Geometry: final body of the model. Coordinates: model frame, mm. Face numbers are marked on the shaded views. A direction names the side the tool comes from. Coordinates: 2 decimals unless noted, no trailing zeros. Write each loop counter-clockwise with the first axis right and the second up, starting at its lowest first coordinate (ties: lowest second). Pieces come first, ordered by that corner, then holes. Notation, with made-up numbers: (81.25, 69) - (117.25, 69) arc R15 ccw to (117.25, 83) - close; hole circle Ø2 at (33.25, -34.5). An arc over 180 degrees is marked (long way). Put each result on its own line as item: value.
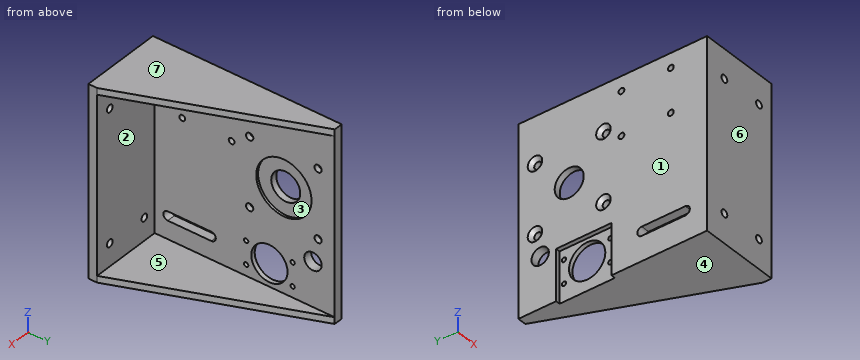
```python
from build123d import *

# Parameters (mm, degrees)
SKETCH1_W                  = 130
SKETCH1_H                  = 130
BOSS_EXTRUDE1_DEPTH        = 6
SKETCH2_W                  = 130
SKETCH2_H                  = 6
BOSS_EXTRUDE2_DEPTH        = 50
BOSS_EXTRUDE3_DEPTH        = 4.5
BOSS_EXTRUDE4_DEPTH        = 4.5
SKETCH5_R                  = 19.05
CUT_EXTRUDE1_DEPTH         = 1.6
SKETCH6_R                  = 10
CUT_EXTRUDE2_DEPTH         = 191.951721647
SKETCH7_R                  = 2.5
CUT_EXTRUDE3_DEPTH         = 193.187408537
SKETCH8_R                  = 12.5
SKETCH8_R_2                = 1.5
ENCODER_MOUNTING_DEPTH     = 193.187408537
SKETCH9_W                  = 35
SKETCH9_H                  = 38
SQR_SLOT_FRO_ENCODER_DEPTH = 3
SKETCH10_R                 = 6
CUT_EXTRUDE6_DEPTH         = 193.187408537
SKETCH12_R                 = 2
CUT_EXTRUDE8_DEPTH         = 193.187408537
CHAMFER1_SIZE              = 2.5
SKETCH14_R                 = 2.5
CUT_EXTRUDE10_DEPTH        = 193.187408537
CUT_EXTRUDE11_DEPTH        = 193.187408537


with BuildPart() as part:
    # Sketch1 → Boss-Extrude1 (new body)
    with BuildSketch(Plane(origin=(0, 0, 0), x_dir=(0, 0, -1), z_dir=(1, 0, 0))):
        with Locations((65, 65)):
            Rectangle(SKETCH1_W, SKETCH1_H)
    extrude(amount=BOSS_EXTRUDE1_DEPTH)

    # Sketch2 → Boss-Extrude2 (add)
    with BuildSketch(Plane(origin=(6, 0, 0), x_dir=(0, 0, -1), z_dir=(1, 0, 0))):
        with Locations((65, 3)):
            Rectangle(SKETCH2_W, SKETCH2_H)
    extrude(amount=BOSS_EXTRUDE2_DEPTH)

    # Sketch3 → Boss-Extrude3 (add)
    with BuildSketch(Plane(origin=(0, 0, -130), x_dir=(-1, 0, 0), z_dir=(0, 0, -1))):
        Polygon((-6, 130), (-56, 6), (-6, 6), align=None)
    extrude(amount=-BOSS_EXTRUDE3_DEPTH)

    # Sketch4 → Boss-Extrude4 (add)
    with BuildSketch(Plane.XY):
        Polygon((6, 130), (56, 6), (6, 6), align=None)
    extrude(amount=-BOSS_EXTRUDE4_DEPTH)

    # Sketch5 → Cut-Extrude1 (cut)
    with BuildSketch(Plane.ZY.offset(-6)):
        with Locations((-55, 95)):
            Circle(SKETCH5_R)
    extrude(amount=CUT_EXTRUDE1_DEPTH, mode=Mode.SUBTRACT)

    # Sketch6 → Cut-Extrude2 (cut, through all)
    with BuildSketch(Plane(origin=(4.4, 0, 0), x_dir=(0, 0, -1), z_dir=(1, 0, 0))):
        with Locations((55, 95)):
            Circle(SKETCH6_R)
    extrude(amount=-CUT_EXTRUDE2_DEPTH, mode=Mode.SUBTRACT)

    # Sketch7 → Cut-Extrude3 (cut, through all)
    with BuildSketch(Plane.ZY):
        with Locations((-78.57, 118.57)):
            Circle(SKETCH7_R)
        with Locations((-31.43, 118.57)):
            Circle(SKETCH7_R)
        with Locations((-31.43, 71.43)):
            Circle(SKETCH7_R)
        with Locations((-78.57, 71.43)):
            Circle(SKETCH7_R)
    extrude(amount=-CUT_EXTRUDE3_DEPTH, mode=Mode.SUBTRACT)

    # Sketch8 → Encoder mounting (cut, through all)
    with BuildSketch(Plane.ZY):
        with Locations((-110, 85)):
            Circle(SKETCH8_R)
        with Locations((-118, 101)):
            Circle(SKETCH8_R_2)
        with Locations((-102, 101)):
            Circle(SKETCH8_R_2)
        with Locations((-102, 69)):
            Circle(SKETCH8_R_2)
        with Locations((-118, 69)):
            Circle(SKETCH8_R_2)
    extrude(amount=-ENCODER_MOUNTING_DEPTH, mode=Mode.SUBTRACT)

    # Sketch9 → Sqr Slot fro encoder (cut)
    with BuildSketch(Plane.ZY):
        with Locations((-112.5, 85)):
            Rectangle(SKETCH9_W, SKETCH9_H)
    extrude(amount=-SQR_SLOT_FRO_ENCODER_DEPTH, mode=Mode.SUBTRACT)

    # Sketch10 → Cut-Extrude6 (cut, through all)
    with BuildSketch(Plane.ZY):
        with Locations((-95, 115)):
            Circle(SKETCH10_R)
    extrude(amount=-CUT_EXTRUDE6_DEPTH, mode=Mode.SUBTRACT)

    # Sketch12 → Cut-Extrude8 (cut, through all)
    with BuildSketch(Plane.ZY):
        with Locations((-10, 25)):
            Circle(SKETCH12_R)
        with Locations((-10, 59)):
            Circle(SKETCH12_R)
        with Locations((-40, 59)):
            Circle(SKETCH12_R)
        with Locations((-40, 25)):
            Circle(SKETCH12_R)
    extrude(amount=-CUT_EXTRUDE8_DEPTH, mode=Mode.SUBTRACT)

    # Chamfer1
    chamfer1_edges = [part.edges().sort_by_distance(p)[0] for p in [
        (0, 118.57, -81.07),
        (0, 118.57, -33.93),
        (0, 71.43, -33.93),
        (0, 71.43, -81.07),
    ]]
    chamfer(chamfer1_edges, length=CHAMFER1_SIZE)

    # Sketch14 → Cut-Extrude10 (cut, through all)
    with BuildSketch(Plane.XZ):
        with Locations(Location((15, -20, 0), (0, 0, 270))):
            Circle(SKETCH14_R)
        with Locations(Location((45, -20, 0), (0, 0, 270))):
            Circle(SKETCH14_R)
        with Locations(Location((15, -110, 0), (0, 0, 270))):
            Circle(SKETCH14_R)
        with Locations(Location((45, -110, 0), (0, 0, 270))):
            Circle(SKETCH14_R)
    extrude(amount=-CUT_EXTRUDE10_DEPTH, mode=Mode.SUBTRACT)

    # Sketch15 → Cut-Extrude11 (cut, through all)
    with BuildSketch(Plane.ZY):
        with BuildLine():
            Line((-113.1, 15), (-113.1, 45))
            ThreePointArc((-113.1, 45), (-110, 48.1), (-106.9, 45))
            Line((-106.9, 45), (-106.9, 15))
            ThreePointArc((-106.9, 15), (-110, 11.9), (-113.1, 15))
        make_face()
    extrude(amount=-CUT_EXTRUDE11_DEPTH, mode=Mode.SUBTRACT)


solid = part.part
```
1. Mould query, pull axis Z, two halves, no side actions, for the marked faces 4, 5, 6 and 7. Classes: +Z half, -Z half, draft (parallel to the pull), parting line (faces both ways), or undercut.
Answer below:
face 4: -Z half
face 5: undercut
face 6: draft
face 7: +Z half
2. Section query C-C (y = 18.5). Return loops of the section in (x, z), then the cut area to 3 significant figures.
Answer below:
outline: (0, -130) - (50.96, -130) - (50.96, -125.5) - (6, -125.5) - (6, -113.1) - (0, -113.1) - close; (0, -106.9) - (6, -106.9) - (6, -4.5) - (50.96, -4.5) - (50.96, 0) - (0, 0) - close
area: 1,150 mm²
3. Section query A-A (z = -10). Return loops of the section in (x, y).
Answer below:
outline: (0, 0) - (56, 0) - (56, 6) - (6, 6) - (6, 23) - (0, 23) - close; (0, 27) - (6, 27) - (6, 57) - (0, 57) - close; (0, 61) - (6, 61) - (6, 130) - (0, 130) - close
4. Set-up query: the marked faces 1, 2 and 3. Return all of +Z, -Z, +X, -X, +Y, -Y with unobstructed straight access to the full face (end or side cutting, diameter ignored); none if empty.
Answer below:
face 1: +Z, -Z, -X, +Y, -Y
face 2: +X, +Y
face 3: +X
5. Section query B-B (x = 27). Return loops of the section in (y, z), then the cut area to 3 significant figures.
Answer below:
outline: (0, -130) - (77.92, -130) - (77.92, -125.5) - (6, -125.5) - (6, -4.5) - (77.92, -4.5) - (77.92, 0) - (0, 0) - close
area: 1,430 mm²
6. Section query D-D (z = -55). Return loops of the section in (x, y).
Answer below:
outline: (0, 0) - (56, 0) - (56, 6) - (6, 6) - (6, 75.95) - (4.4, 75.95) - (4.4, 85) - (0, 85) - close; (0, 105) - (4.4, 105) - (4.4, 114.05) - (6, 114.05) - (6, 130) - (0, 130) - close
7. Ray query, probe 1 along Y at (x, z) = (4.45, -78.57); probe 2 along Z at (x, y) = (9, 31); probe 3 along Y at (x, z) = (3.3, -55). Return the intervals inside material, ascending. Write a range as from..to.
Answer below:
probe 1: y = 0..68.93, 73.93..116.07, 121.07..130
probe 2: z = -130..-125.5, -4.5..0
probe 3: y = 0..85, 105..130
8. Pin query (flat end, axial travel): pin 1 Ø0.9 at (x, y) = (1, 89.5) entering from -Z; pin 2 Ø15.5 at (y, z) = (115, -95) entering from +X; pin 3 Ø17.5 at (y, z) = (78, -110) entering from -X. Return the tip coordinate at first contact, or that it passes through.
Answer below:
pin 1: stops at z = -95
pin 2: stops at x = 6
pin 3: stops at x = 3
